Geometry check sheet. Reference: the model listing, model coordinates, mm. A direction names the side the tool comes from. Round coordinates to 2 decimals unless told otherwise and drop trailing zeros. Order: outer loops, then holes, each group sorted by start corner. A loop starts at its lowest first (then second) coordinate and runs counter-clockwise, first axis right, second up. Notation, with made-up numbers: (-14.75, -23) - (7.25, -23) arc R12 ccw to (7.25, -10) - close; hole circle Ø4 at (28, 33.25). An arc over 180 degrees is marked (long way). Answer as CSV lines item,"result". Start each with the question number.
Autodesk Inventor part; units mm, degrees
ref_plane "YZ Plane" through (0, 0, 0) normal (1, 0, 0) x (0, 1, 0)
ref_plane "XZ Plane" through (0, 0, 0) normal (0, 1, 0) x (-1, 0, 0)
ref_plane "XY Plane" through (0, 0, 0) normal (0, 0, 1) x (1, 0, 0)
sketch "Sketch1" plane through (0, 0, 0) normal (0, 1, 0) x (-1, 0, 0)
  line L0 (0, 0) -> (13, 0)
  line L1 (13, 0) -> (13, -19)
  line L2 (13, -19) -> (0, -19)
  line L3 (0, -19) -> (0, 0)
  line L4 (0, 0) -> (-3, 0)
  line L5 (-3, 0) -> (-3, 3)
  line L6 (-3, 3) -> (0, 3)
  line L7 (0, 3) -> (0, 0)
  line L8 (13, -19) -> (16, -19)
  line L9 (16, -19) -> (16, -22)
  line L10 (16, -22) -> (13, -22)
  line L11 (13, -22) -> (13, -19)
  line L12 (16, -22) -> (-3, -22)
  line L13 (-3, -22) -> (-3, 3)
  line L14 (-3, 3) -> (16, 3)
  line L15 (16, 3) -> (16, -22)
  dimension "d0" = 13
  dimension "d1" = 19
  dimension "d2" = 3
  dimension "d3" = 3
  dimension "d4" = 3
  dimension "d5" = 3
extrude "Extrusion1" add sketch "Sketch1" along normal blind 4 contours L7 L14 L15 L8 L1 L0 | L3 L2 L11 L12 L13 L4 | L4 L5 L6 L7 | L8 L9 L10 L11
sketch "Sketch2" plane through (3, 0, 3) normal (1, 0, 0) x (0, 0, -1)
  line L0 (25, 0) -> (25, 4)
  line L1 (25, 0) -> (0, 0)
  line L2 (25, 0) -> (0, 0)
  line L3 (25, 0) -> (12.5, 0)
  line L4 (3, 0) -> (22, 0)
  line L5 (12.5, 0) -> (12.5, -4)
  circle A0 centre (12.5, -4) radius 1.5
  line L6 (12.5, -4) -> (22.5, -4)
  line L7 (22.5, -4) -> (2.5, -4)
  circle A1 centre (2.5, -4) radius 1.5
  circle A2 centre (22.5, -4) radius 1.5
  line L8 (0, 0) -> (25, 0)
  line L9 (25, 0) -> (25, -7)
  line L10 (25, -7) -> (0, -7)
  line L11 (0, -7) -> (0, 0)
  line L12 (25, 0) -> (25, 4)
  line L13 (0, 0) -> (25, 0)
  line L14 (25, 0) -> (25, 4)
  line L15 (25, 4) -> (0, 4)
  line L16 (0, 4) -> (0, 0)
  dimension "d8" = 12.5
  dimension "d9" = 4
  dimension "d10" = 3
  dimension "d11" = 10
  dimension "d12" = 20
  dimension "d13" = 3
  dimension "d14" = 3
  dimension "d15" = 7
extrude "Extrusion2" add sketch "Sketch2" along normal mid plane 6
fillet "Fillet1" radius 2 4 edges at (-16, 2, -22) (-16, 2, 3) (3, -7, 3) (3, -7, -22)
fillet "Fillet2" radius 2 2 edges at (0, 0, -20.5) (0, 0, 1.5)
sketch "Sketch3" plane through (0, 4, 0) normal (0, 1, 0) x (1, 0, 0)
  point P0 (0, 0)
properties part number "power_button_holder"
1. Section check B-B on z = -19.5. Record the boundary of the cut face in (x, y), plus the area to 3 significant figures.
2. Section check C-C on y = -4. Record the boundary of the cut face in (x, z).
3. Section check A-A on x = -5.5. Record the boundary of the cut face in (y, z).
4. Access from +Z, -Z, +X, -X, +Y, -Y to the whole of each face (thin tool, end or side, straight path). Record for faces 5 (the face through (-14, 0, -9)), 6 (the face through (-15.4, 2.03, -21.43)), 7 (the face through (-6, 2, 0)).
5. Thickness scan on probe 1 along Y at (x, z) = (3.5, -9.5); probe 2 along Z at (x, y) = (3.5, -4.5); probe 3 along Z at (x, y) = (-2.25, 3). Record the ranges inside material, lowest first.
6. Section check D-D on x = 1.25. Record the boundary of the cut face in (y, z).
7. Draft check along Y on faces 1 (the face through (3, -4, -18)), 2 (the face through (0, -1, -9)), 3 (the face through (3, -7, -10)), 4 (the face through (2, 4, -9)). Enter one of: released by +Y, released by -Y, zero draft, split by the parting line, or undercut.
Numbers:
1,outline,"(-16, 0) - (-2, 0) arc R2 cw to (0, -2) - (0, -2.5) - (6, -2.5) - (6, 4) - (-16, 4) - close; (0, -7) - (6, -7) - (6, -5.5) - (0, -5.5) - close"
1,area,"113 mm2"
2,outline,"(0, -22) - (6, -22) - (6, -21) - (0, -21) - close; (0, -18) - (6, -18) - (6, -11) - (0, -11) - close; (0, -8) - (6, -8) - (6, -1) - (0, -1) - close; (0, 2) - (6, 2) - (6, 3) - (0, 3) - close"
3,outline,"(0, -22) - (4, -22) - (4, -19) - (0, -19) - close; (0, 0) - (4, 0) - (4, 3) - (0, 3) - close"
4,face 5,"+Z, -Z, -X, -Y"
4,face 6,"-Z, -X, +Y, -Y"
4,face 7,"+Y, -Y"
5,probe 1,"y = -7 to -5.5, -2.5 to 4"
5,probe 2,"z = -22 to -20.91, -18.09 to -10.91, -8.09 to -0.91, 1.91 to 3"
5,probe 3,"z = -22 to -19, 0 to 3"
6,outline,"(-7, -20) arc R2 ccw to (-5, -22) - (4, -22) - (4, 3) - (-5, 3) arc R2 ccw to (-7, 1) - close; hole circle Ø3 at (-4, -19.5); hole circle Ø3 at (-4, -9.5); hole circle Ø3 at (-4, 0.5)"
7,face 1,"undercut"
7,face 2,"zero draft"
7,face 3,"released by -Y"
7,face 4,"released by +Y"
